Could you check a few things on this drawing? It's one solid part, dimensions in mm from its lowest x, y, z. A direction names the side the tool comes from. Round coordinates to 2 decimals unless told otherwise and drop trailing zeros. Order: outer loops, then holes, each group sorted by start corner. A loop starts at its lowest first (then second) coordinate and runs counter-clockwise, first axis right, second up.
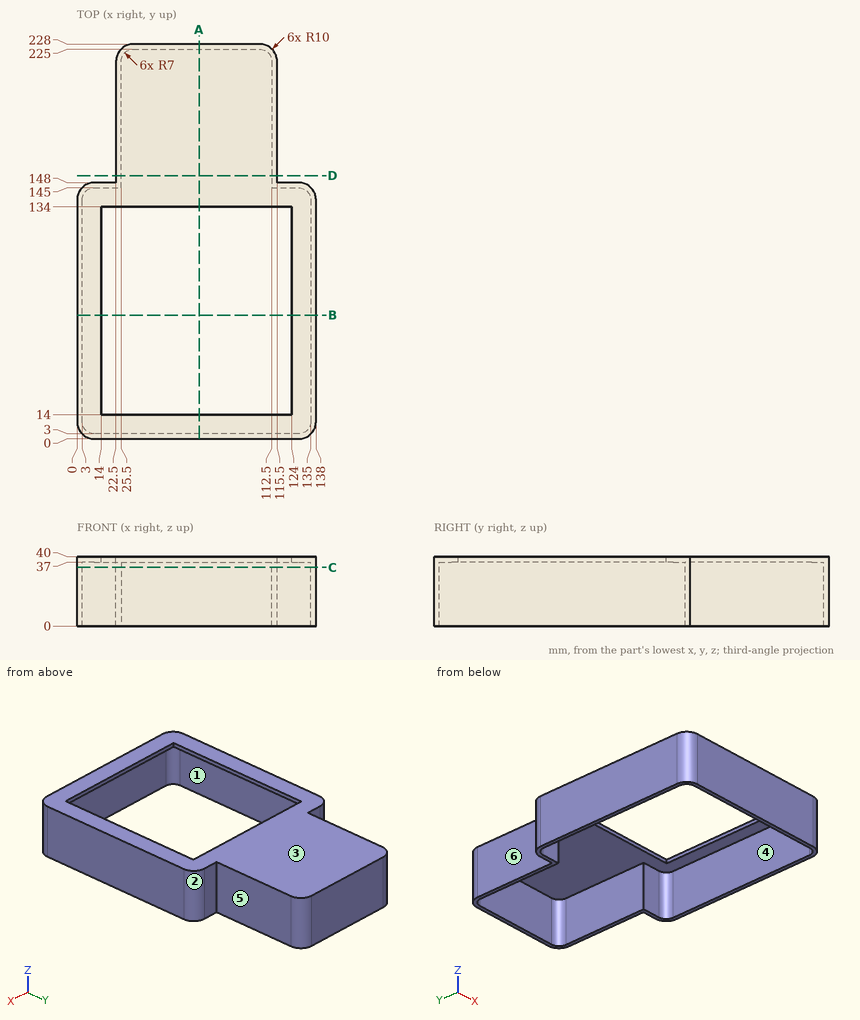
(1) I want a section at D-D, the plane y = 152. List the corners of the cut face in (x, z) for me.
(2) If we mould it in two halves opening along X, with no side actions, what happens to the marked faces 1, 2 and 3? For each: pulls with the +X half, pulls with the -X half, needs draft (parallel to the pull), parting line crosses it, or undercut.
(3) Please list where these lines run through material, in increasing order: probe 1 along X at (y, z) = (12.5, 12); probe 2 along Y at (x, z) = (98.5, 3.5); probe 3 along Y at (x, z) = (12, 2).
(4) I'm going to push flat-ended pins straight in: pin 1 Ø1.5 at (y, z) = (172.5, 16) entering from +X; pin 2 Ø4 at (x, z) = (29.5, 30.5) entering from +Y; pin 3 Ø6 at (x, z) = (116, 4) entering from +Y. Where does each tip first touch, or does it pass through?
(5) I want a section at B-B, the plane y = 71.5. List the corners of the cut face in (x, z) for me.
(6) I want a section at A-A, the plane x = 70.5. List the corners of the cut face in (y, z) for me.
(7) I want a section at C-C, the plane z = 34. List the corners of the cut face in (x, y) for me.
(8) On a 3-axis mill with a long thin cutter (end or side, diameter ignored), from which of +Z, -Z, +X, -X, +Y, -Y can I reach the whole of each face in a straight line? I mean the marked faces 4, 5 and 6. Say none if no direction works.
Ans:
1. outline: (22.5, 0) - (25.5, 0) - (25.5, 37) - (112.5, 37) - (112.5, 0) - (115.5, 0) - (115.5, 40) - (22.5, 40) - close
2. face 1: undercut
2. face 2: pulls with the +X half
2. face 3: needs draft
3. probe 1: x = 0 to 3, 135 to 138
3. probe 2: y = 0 to 3, 225 to 228
3. probe 3: y = 0 to 3, 145 to 148
4. pin 1: stops at x = 115.5
4. pin 2: stops at y = 227.95
4. pin 3: stops at y = 224.61
5. outline: (0, 0) - (3, 0) - (3, 37) - (14, 37) - (14, 40) - (0, 40) - close; (124, 37) - (135, 37) - (135, 0) - (138, 0) - (138, 40) - (124, 40) - close
6. outline: (0, 0) - (3, 0) - (3, 37) - (14, 37) - (14, 40) - (0, 40) - close; (134, 37) - (225, 37) - (225, 0) - (228, 0) - (228, 40) - (134, 40) - close
7. outline: (0, 10) arc R10 ccw to (10, 0) - (128, 0) arc R10 ccw to (138, 10) - (138, 138) arc R10 ccw to (128, 148) - (115.5, 148) - (115.5, 218) arc R10 ccw to (105.5, 228) - (32.5, 228) arc R10 ccw to (22.5, 218) - (22.5, 148) - (10, 148) arc R10 ccw to (0, 138) - close; hole (3, 10) arc R7 ccw to (10, 3) - (128, 3) arc R7 ccw to (135, 10) - (135, 138) arc R7 ccw to (128, 145) - (112.5, 145) - (112.5, 218) arc R7 ccw to (105.5, 225) - (32.5, 225) arc R7 ccw to (25.5, 218) - (25.5, 145) - (10, 145) arc R7 ccw to (3, 138) - close
8. face 4: -Z
8. face 5: +Z, -Z, +X, +Y
8. face 6: +Z, -Z, -X, +Y
